Geometry check sheet. Reference: the model listing, model coordinates, mm. A direction names the side the tool comes from. Coordinates: 2 decimals unless noted, no trailing zeros. Write each loop counter-clockwise with the first axis right and the second up, starting at its lowest first coordinate (ties: lowest second). Pieces come first, ordered by that corner, then holes. Notation, with made-up numbers: (-39.75, 0) -> (12.25, 0) arc R15 ccw to (12.25, 21) -> close; hole circle Ø2 at (4.25, -20.75). An arc over 180 degrees is marked (long way). Use a Markdown table: item, result.
```python
from build123d import *

# Parameters (mm, degrees)
BOSS_EXTRUDE1_DEPTH = 20
SKETCH3_W           = 76
SKETCH3_H           = 2
BOSS_EXTRUDE2_DEPTH = 30
FILLET2_R           = 1
FILLET3_R           = 0.5
SKETCH4_W           = 3
SKETCH4_H           = 62
BOSS_EXTRUDE3_DEPTH = 10
SKETCH5_W           = 76
SKETCH5_H           = 8
BOSS_EXTRUDE4_DEPTH = 1
FILLET5_R           = 2


with BuildPart() as part:
    # Sketch1 → Boss-Extrude1 (new body)
    with BuildSketch(Plane(origin=(0, 0, 0), x_dir=(0, 1, 0), z_dir=(0, 0, 1))):
        Polygon((-38.603475532, 1.8), (-41.25, 1.8), (-41.25, -3.8), (41.25, -3.8), (41.25, 1.8), (38.603475532, 1.8), (38.603475532, 0.8), (40.25, 0.8), (40.25, -0.8), (-38.603475532, -0.8), (-40.25, -0.8), (-40.25, 0.8), (-38.603475532, 0.8), align=None)
    extrude(amount=BOSS_EXTRUDE1_DEPTH)

    # Sketch3 → Boss-Extrude2 (add)
    with BuildSketch(Plane.XY.offset(20)):
        with Locations((38.8, 0)):
            Rectangle(SKETCH3_W, SKETCH3_H)
    extrude(amount=-BOSS_EXTRUDE2_DEPTH)

    # Fillet2
    fillet2_edges = [part.edges().sort_by_distance(p)[0] for p in [
        (3.8, 41.25, 10),
        (3.8, -41.25, 10),
    ]]
    fillet(fillet2_edges, radius=FILLET2_R)

    # Fillet3
    fillet3_edges = [part.edges().sort_by_distance(p)[0] for p in [
        (-1.8, 41.25, 10),
        (-1.8, -41.25, 10),
    ]]
    fillet(fillet3_edges, radius=FILLET3_R)

    # Sketch4 → Boss-Extrude3 (add)
    with BuildSketch(Plane(origin=(0, 0, 0), x_dir=(1, 0, 0), z_dir=(0, 0, -1))):
        with Locations((2.3, 0)):
            Rectangle(SKETCH4_W, SKETCH4_H)
    extrude(amount=BOSS_EXTRUDE3_DEPTH)

    # Sketch5 → Boss-Extrude4 (add)
    with BuildSketch(Plane(origin=(0, 0, -10), x_dir=(1, 0, 0), z_dir=(0, 0, -1))):
        with Locations((38.8, 0)):
            Rectangle(SKETCH5_W, SKETCH5_H)
    extrude(amount=-BOSS_EXTRUDE4_DEPTH)

    # Fillet5
    fillet5_edges = [part.edges().sort_by_distance(p)[0] for p in [
        (3.8, -1, 5.5),
        (40.3, 1, -9),
        (40.3, -1, -9),
        (3.8, 1, 5.5),
    ]]
    fillet(fillet5_edges, radius=FILLET5_R)


solid = part.part
```
Item 1: Section check B-B on x = 25. Record the boundary of the cut face in (y, z), then the cut area to 3 significant figures.
Answer block:
| item | result |
|---|---|
| outline | (-4, -10) -> (4, -10) -> (4, -9) -> (3, -9) arc R2 cw to (1, -7) -> (1, 20) -> (-1, 20) -> (-1, -7) arc R2 cw to (-3, -9) -> (-4, -9) -> close |
| area | 67.7 mm^2 |
Item 2: Tool access check on faces 1 (the flat face through (41, 1, 7)), 2 (the flat face through (41, -1, 7)), 3 (the flat face through (2, 31, -5)). Record the directions out of +Z, -Z, +X, -X, +Y, -Y that give a thin tool (end or side, any length) a straight path to the whole face; none if there is none.
Answer block:
| item | result |
|---|---|
| face 1 | +Z, +X, +Y |
| face 2 | +Z, +X, -Y |
| face 3 | -Z, +X, -X, +Y |
Item 3: Mould release check, pull along Y, two halves, no side actions. Record for faces 4 (the flat face through (0.8, 1, 5)), 5 (the flat face through (3.8, -22, 5)), 6 (the flat face through (1, 41.25, 10)), 7 (the cylindrical face through (4.37, -1.6, 5.7)): +Y half, -Y half, draft (parallel to the pull), parting line (faces both ways), or undercut.
Answer block:
| item | result |
|---|---|
| face 4 | undercut |
| face 5 | draft |
| face 6 | +Y half |
| face 7 | -Y half |
Item 4: Thickness scan on L1, parallel to Y at x = 8, z = -2.25; L2, parallel to X at y = 10, z = -1.5; L3, parallel to X at y = -1.5, z = 10. Record the ranges inside material, lowest first. Write a range as [from, to].
Answer block:
| item | result |
|---|---|
| L1 | y = [-1, 1] |
| L2 | x = [0.8, 3.8] |
| L3 | x = [0.8, 4.48] |
Item 5: Section check C-C on y = -32. Record the boundary of the cut face in (x, z).
Answer block:
| item | result |
|---|---|
| outline | (0.8, 0) -> (3.8, 0) -> (3.8, 20) -> (0.8, 20) -> close |
Item 6: Section check A-A on z = -3.5. Record the boundary of the cut face in (x, y), then the cut area to 3 significant figures.
Answer block:
| item | result |
|---|---|
| outline | (0.8, -31) -> (3.8, -31) -> (3.8, -3) arc R2 cw to (5.8, -1) -> (76.8, -1) -> (76.8, 1) -> (5.8, 1) arc R2 cw to (3.8, 3) -> (3.8, 31) -> (0.8, 31) -> close |
| area | 334 mm^2 |
Item 7: Section check D-D on z = 15.75. Record the boundary of the cut face in (x, y).
Answer block:
| item | result |
|---|---|
| outline | (-1.8, -40.75) arc R0.5 ccw to (-1.3, -41.25) -> (2.8, -41.25) arc R1 ccw to (3.8, -40.25) -> (3.8, -3) arc R2 cw to (5.8, -1) -> (76.8, -1) -> (76.8, 1) -> (5.8, 1) arc R2 cw to (3.8, 3) -> (3.8, 40.25) arc R1 ccw to (2.8, 41.25) -> (-1.3, 41.25) arc R0.5 ccw to (-1.8, 40.75) -> (-1.8, 38.6) -> (-0.8, 38.6) -> (-0.8, 40.25) -> (0.8, 40.25) -> (0.8, -40.25) -> (-0.8, -40.25) -> (-0.8, -38.6) -> (-1.8, -38.6) -> close |
Item 8: Depth check by flat-ended pin: P1, Ø3.5, axis at x = 3, z = -7.5, coming from the +Y side; P2, Ø4.5, axis at x = 1, y = 36.5, coming from the -Z side; P3, Ø1.1, axis at x = 33, y = -3.5, coming from the +Z side. Enter the tip coordinate at first touch or a pass-through.
Answer block:
| item | result |
|---|---|
| P1 | stops at y = 31 |
| P2 | stops at z = 0 |
| P3 | stops at z = -9 |
